Autodesk Inventor part; units mm, degrees
ref_plane "YZ Plane" through (0, 0, 0) normal (1, 0, 0) x (0, 1, 0)
ref_plane "XZ Plane" through (0, 0, 0) normal (0, 1, 0) x (-1, 0, 0)
ref_plane "XY Plane" through (0, 0, 0) normal (0, 0, 1) x (1, 0, 0)
sketch "Náčrt1" plane through (0, 0, 0) normal (0, 0, 1) x (1, 0, 0)
  line L0 (-10, 0) -> (0, 0)
  line L1 (0, 0) -> (0, 20)
  line L2 (0, 20) -> (-1.5, 20)
  line L3 (-1.5, 20) -> (-1.5, 1.5)
  line L4 (-1.5, 1.5) -> (-10, 1.5)
  line L5 (-10, 1.5) -> (-10, 0)
  line L6 (-12, 0) -> (2, 0)
  line L7 (0, 24) -> (0, -4)
  point P0 (0, 0)
  dimension "d0" = 20
  dimension "d1" = 10
  dimension "d2" = 1.5
  dimension "d3" = 1.5
extrude "Vysunutí1" add sketch "Náčrt1" along normal mid plane 45
sketch "Náčrt2" plane through (-10, 1.5, 22.5) normal (0, 1, 0) x (1, 0, 0)
  line L0 (0, 0) -> (0, 45)
  line L1 (8.5, 0) -> (0, 0)
  line L2 (8.5, 45) -> (8.5, 0)
  line L3 (0, 45) -> (8.5, 45)
  point P0 (10, 22.5)
  point P1 (4.25, 35)
  point P2 (4.25, 10)
  point P3 (4.25, 0)
  dimension "d6" = 4.25
  dimension "d7" = 4.25
  dimension "d8" = 25
  dimension "d9" = 10
hole "Díra1" at (-5.75, 1.5, -12.5) at (-5.75, 1.5, 12.5) direction (0, -1, 0) diameter 4.5 end through all
sketch "Náčrt3" plane through (-1.5, 1.5, 22.5) normal (-1, 0, 0) x (0, 0, 1)
  line L0 (-45, 0) -> (0, 0)
  line L1 (0, 18.5) -> (0, 0)
  line L2 (-45, 18.5) -> (0, 18.5)
  line L3 (-45, 0) -> (-45, 18.5)
  point P0 (-22.5, -1.5)
  point P1 (-12, 13.5)
  point P2 (-22, 13.5)
  dimension "d17" = 10
  dimension "d18" = 5
  dimension "d19" = 5
  dimension "d20" = 12
hole "Díra2" at (-1.5, 15, 10.5) at (-1.5, 15, 0.5) direction (1, 0, 0) diameter 3.2 end through all
sketch "Náčrt4" plane through (-1.5, 1.5, 22.5) normal (-1, 0, 0) x (0, 0, 1)
  circle A0 centre (-22, 13.5) radius 1.6
  circle A1 centre (-12, 13.5) radius 1.6
  line L0 (-45, 0) -> (0, 0)
  line L1 (0, 18.5) -> (0, 0)
  line L2 (-45, 18.5) -> (0, 18.5)
  line L3 (-45, 0) -> (-45, 18.5)
  line L4 (-45, -1.5) -> (0, -1.5)
  point P0 (-22.5, -1.5)
  point P1 (-30, 3.5)
  point P2 (-12, 3.5)
  dimension "d28" = 5
  dimension "d29" = 5
  dimension "d30" = 18
  dimension "d31" = 12
hole "Díra3" at (-1.5, 5, -7.5) at (-1.5, 5, 10.5) direction (1, 0, 0) diameter 2.459 end through all
properties part number "x_bracket" material "Hliník 6061"
Check sheet for the modelled part. Datum: model origin and axes. Units: mm. A direction names the side the tool comes from. Coordinates: 2 decimals unless noted, no trailing zeros. Write each loop counter-clockwise with the first axis right and the second up, starting at its lowest first coordinate (ties: lowest second). Pieces come first, ordered by that corner, then holes.
Item 1: Cross-section at B-B on x = -5.75. Record the boundary of the cut face in (y, z), then the cut area to 3 significant figures.
Numbers:
outline: (0, -22.5) - (1.5, -22.5) - (1.5, -14.75) - (0, -14.75) - close; (0, -10.25) - (1.5, -10.25) - (1.5, 10.25) - (0, 10.25) - close; (0, 14.75) - (1.5, 14.75) - (1.5, 22.5) - (0, 22.5) - close
area: 54.0 mm2
Item 2: Depth check by flat-ended pin: pin 1 Ø1 at (y, z) = (5.5, -10.5) entering from -X; pin 2 Ø1 at (x, z) = (-1.5, -7) entering from -Y; pin 3 Ø4 at (x, z) = (-5.5, 10.5) entering from +Y. Enter the tip coordinate at first touch or a pass-through.
Numbers:
pin 1: stops at x = -1.5
pin 2: stops at y = 0
pin 3: stops at y = 1.5
Item 3: Cross-section at C-C on z = 7. Record the boundary of the cut face in (x, y).
Numbers:
outline: (-10, 0) - (0, 0) - (0, 20) - (-1.5, 20) - (-1.5, 1.5) - (-10, 1.5) - close
Item 4: Access from +Z, -Z, +X, -X, +Y, -Y to the whole of each face (thin tool, end or side, straight path). Record for faces 4 (the face through (-1, 20, 0)), 5 (the face through (-6, 1.5, 0)).
Numbers:
face 4: +Z, -Z, +X, -X, +Y
face 5: +Z, -Z, -X, +Y
Item 5: Cross-section at A-A on z = 0.5. Record the boundary of the cut face in (x, y), then the cut area to 4 significant figures.
Numbers:
outline: (-10, 0) - (0, 0) - (0, 13.4) - (-1.5, 13.4) - (-1.5, 1.5) - (-10, 1.5) - close; (-1.5, 16.6) - (0, 16.6) - (0, 20) - (-1.5, 20) - close
area: 37.95 mm2
Item 6: Cross-section at D-D on z = -7.5. Record the boundary of the cut face in (x, y).
Numbers:
outline: (-10, 0) - (0, 0) - (0, 3.77) - (-1.5, 3.77) - (-1.5, 1.5) - (-10, 1.5) - close; (-1.5, 6.23) - (0, 6.23) - (0, 20) - (-1.5, 20) - close
Item 7: Mould release check, pull along Z, two halves, no side actions. Record for faces 1 (the face through (-1, 7, -22.5)), 2 (the face through (-0.74, 5.471, 11.636)), 3 (the face through (-10, 1, 0)): released by +Z, released by -Z, zero draft, split by the parting line, or undercut.
Numbers:
face 1: released by -Z
face 2: undercut
face 3: zero draft
Item 8: Scan lines: probe 1 along Y at (x, z) = (-0.7, 10.5); probe 2 along Z at (x, y) = (-5.75, 0.8); probe 3 along Z at (x, y) = (-0.6, 15). Record each from-to range of solid material in increasing order.
Numbers:
probe 1: y = 0 to 3.77, 6.23 to 13.4, 16.6 to 20
probe 2: z = -22.5 to -14.75, -10.25 to 10.25, 14.75 to 22.5
probe 3: z = -22.5 to -1.1, 2.1 to 8.9, 12.1 to 22.5
